Check sheet for the modelled part. Datum: model origin and axes. Units: mm. Give positions to 0.01 mm unless a question says otherwise; leave off trailing zeros. Write each loop counter-clockwise with the first axis right and the second up, starting at its lowest first coordinate (ties: lowest second). Pieces come first, ordered by that corner, then holes. Notation, with made-up numbers: (36, -5.5) -> (62, -5.5) arc R16 ccw to (62, 15.5) -> close; hole circle Ø2 at (64, 48). An arc over 180 degrees is marked (long way). Return JSON: item names as keys, results as strings.
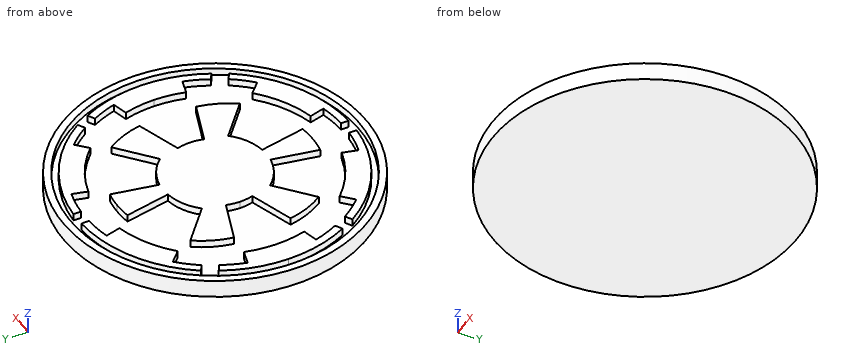
from build123d import *

# Parameters (mm, degrees)
F2_R     = 53.34
F3_DEPTH = 6.35
F0_R     = 50.8
F4_DEPTH = 2.54
F5_DEPTH = 2.54


with BuildPart() as f3:
    # F2 (on Top) → F3 (new body)
    with BuildSketch(Plane.XY):
        Circle(F2_R)
    extrude(amount=-F3_DEPTH)

    # F0 (on Top) → F4 (cut)
    with BuildSketch(Plane.XY):
        Circle(F0_R)
    extrude(amount=-F4_DEPTH, mode=Mode.SUBTRACT)

    # F1 (on Top) → F5 (join)
    with BuildSketch(Plane.XY):
        with BuildLine():
            ThreePointArc((-43.063388, 21.784679), (-46.942873, 11.197957), (-48.26, 0))
            ThreePointArc((-48.26, 0), (-46.942873, -11.197957), (-43.063388, -21.784679))
            Line((-43.063388, -21.784679), (-40.692139, -20.398091))
            ThreePointArc((-40.692139, -20.398091), (-42.512578, -16.297657), (-43.915142, -12.036159))
            Line((-43.915142, -12.036159), (-38.702908, -10.612585))
            ThreePointArc((-38.702908, -10.612585), (-39.772793, -5.354158), (-40.13156, 0))
            ThreePointArc((-40.13156, 0), (-39.772793, 5.354158), (-38.702908, 10.612585))
            Line((-38.702908, 10.612585), (-43.915142, 12.036159))
            ThreePointArc((-43.915142, 12.036159), (-42.512578, 16.297657), (-40.692139, 20.398091))
            Line((-40.692139, 20.398091), (-43.063388, 21.784679))
        make_face()
        with BuildLine():
            Line((-38.165818, -25.239456), (-40.531515, -26.604988))
            ThreePointArc((-40.531515, -26.604988), (-24.179309, -42.023686), (-2.631168, -48.411839))
            Line((-2.631168, -48.411839), (-2.631168, -45.742772))
            ThreePointArc((-2.631168, -45.742772), (-7.132062, -45.269114), (-11.555377, -44.311676))
            Line((-11.555377, -44.311676), (-10.181512, -39.106512))
            ThreePointArc((-10.181512, -39.106512), (-20.139594, -35.033973), (-28.670142, -28.478157))
            Line((-28.670142, -28.478157), (-32.500429, -32.26304))
            ThreePointArc((-32.500429, -32.26304), (-35.517393, -28.899884), (-38.165818, -25.239456))
        make_face()
        with BuildLine():
            Line((-2.71646, -18.05863), (-5.79492, -33.915079))
            ThreePointArc((-5.79492, -33.915079), (-2.907863, -34.283495), (0, -34.406594))
            ThreePointArc((0, -34.406594), (2.907863, -34.283495), (5.79492, -33.915079))
            Line((5.79492, -33.915079), (2.71646, -18.05863))
            ThreePointArc((2.71646, -18.05863), (8.779304, -16.013029), (13.764323, -12.001529))
            Line((13.764323, -12.001529), (25.921796, -22.591443))
            ThreePointArc((25.921796, -22.591443), (29.145002, -16.549346), (31.013678, -9.961172))
            Line((31.013678, -9.961172), (15.781759, -4.649021))
            ThreePointArc((15.781759, -4.649021), (16.283782, -2.348563), (16.452274, 0))
            ThreePointArc((16.452274, 0), (16.283782, 2.348563), (15.781759, 4.649021))
            Line((15.781759, 4.649021), (31.013678, 9.961172))
            ThreePointArc((31.013678, 9.961172), (29.145002, 16.549346), (25.921796, 22.591443))
            Line((25.921796, 22.591443), (13.764323, 12.001529))
            ThreePointArc((13.764323, 12.001529), (8.779304, 16.013029), (2.71646, 18.05863))
            Line((2.71646, 18.05863), (5.79492, 33.915079))
            ThreePointArc((5.79492, 33.915079), (2.907863, 34.283495), (0, 34.406594))
            ThreePointArc((0, 34.406594), (-2.907863, 34.283495), (-5.79492, 33.915079))
            Line((-5.79492, 33.915079), (-2.71646, 18.05863))
            ThreePointArc((-2.71646, 18.05863), (-8.779304, 16.013029), (-13.764323, 12.001529))
            Line((-13.764323, 12.001529), (-25.921796, 22.591443))
            ThreePointArc((-25.921796, 22.591443), (-29.145002, 16.549346), (-31.013678, 9.961172))
            Line((-31.013678, 9.961172), (-15.781759, 4.649021))
            ThreePointArc((-15.781759, 4.649021), (-16.283782, 2.348563), (-16.452274, 0))
            ThreePointArc((-16.452274, 0), (-16.283782, -2.348563), (-15.781759, -4.649021))
            Line((-15.781759, -4.649021), (-31.013678, -9.961172))
            ThreePointArc((-31.013678, -9.961172), (-29.145002, -16.549346), (-25.921796, -22.591443))
            Line((-25.921796, -22.591443), (-13.764323, -12.001529))
            ThreePointArc((-13.764323, -12.001529), (-8.779304, -16.013029), (-2.71646, -18.05863))
        make_face()
        with BuildLine():
            Line((2.631168, -45.742772), (2.631168, -48.411839))
            ThreePointArc((2.631168, -48.411839), (24.179309, -42.023686), (40.531515, -26.604988))
            Line((40.531515, -26.604988), (38.165818, -25.239456))
            ThreePointArc((38.165818, -25.239456), (35.517393, -28.899884), (32.500429, -32.26304))
            Line((32.500429, -32.26304), (28.670142, -28.478157))
            ThreePointArc((28.670142, -28.478157), (20.139594, -35.033973), (10.181512, -39.106512))
            Line((10.181512, -39.106512), (11.555377, -44.311676))
            ThreePointArc((11.555377, -44.311676), (7.132062, -45.269114), (2.631168, -45.742772))
        make_face()
        with BuildLine():
            ThreePointArc((40.13156, 0), (39.772793, -5.354158), (38.702908, -10.612585))
            Line((38.702908, -10.612585), (43.915142, -12.036159))
            ThreePointArc((43.915142, -12.036159), (42.512578, -16.297657), (40.692139, -20.398091))
            Line((40.692139, -20.398091), (43.063388, -21.784679))
            ThreePointArc((43.063388, -21.784679), (46.942873, -11.197957), (48.26, 0))
            ThreePointArc((48.26, 0), (46.942873, 11.197957), (43.063388, 21.784679))
            Line((43.063388, 21.784679), (40.692139, 20.398091))
            ThreePointArc((40.692139, 20.398091), (42.512578, 16.297657), (43.915142, 12.036159))
            Line((43.915142, 12.036159), (38.702908, 10.612585))
            ThreePointArc((38.702908, 10.612585), (39.772793, 5.354158), (40.13156, 0))
        make_face()
        with BuildLine():
            ThreePointArc((40.531515, 26.604988), (24.179309, 42.023686), (2.631168, 48.411839))
            Line((2.631168, 48.411839), (2.631168, 45.742772))
            ThreePointArc((2.631168, 45.742772), (7.132062, 45.269114), (11.555377, 44.311676))
            Line((11.555377, 44.311676), (10.181512, 39.106512))
            ThreePointArc((10.181512, 39.106512), (20.139594, 35.033973), (28.670142, 28.478157))
            Line((28.670142, 28.478157), (32.500429, 32.26304))
            ThreePointArc((32.500429, 32.26304), (35.517393, 28.899884), (38.165818, 25.239456))
            Line((38.165818, 25.239456), (40.531515, 26.604988))
        make_face()
        with BuildLine():
            ThreePointArc((-2.631168, 48.411839), (-24.179309, 42.023686), (-40.531515, 26.604988))
            Line((-40.531515, 26.604988), (-38.165818, 25.239456))
            ThreePointArc((-38.165818, 25.239456), (-35.517393, 28.899884), (-32.500429, 32.26304))
            Line((-32.500429, 32.26304), (-28.670142, 28.478157))
            ThreePointArc((-28.670142, 28.478157), (-20.139594, 35.033973), (-10.181512, 39.106512))
            Line((-10.181512, 39.106512), (-11.555377, 44.311676))
            ThreePointArc((-11.555377, 44.311676), (-7.132062, 45.269114), (-2.631168, 45.742772))
            Line((-2.631168, 45.742772), (-2.631168, 48.411839))
        make_face()
    extrude(amount=-F5_DEPTH)


solid = f3.part
(1) Thickness scan on L1, parallel to X at y = 22, z = -1; L2, parallel to Y at x = -41, z = -1; L3, parallel to Z at x = 39, y = -19. Record the ranges inside material, lowest first.
Reply:
{"L1": "-48.59 to -45.79, -26.31 to -25.24, -3.48 to 3.48, 25.24 to 26.31, 45.79 to 48.59", "L2": "-34.12 to -29.99, -20.58 to -19.78, -11.24 to 11.24, 19.78 to 20.58, 29.99 to 34.12", "L3": "-6.35 to -2.54"}
(2) Cross-section at D-D on y = 6. Enter the section's corners in (x, z), then the cut area to 3 significant figures.
Reply:
{"outline": "(-53, -6.35) -> (53, -6.35) -> (53, 0) -> (50.44, 0) -> (50.44, -2.54) -> (47.89, -2.54) -> (47.89, 0) -> (39.68, 0) -> (39.68, -2.54) -> (19.66, -2.54) -> (19.66, 0) -> (-19.66, 0) -> (-19.66, -2.54) -> (-39.68, -2.54) -> (-39.68, 0) -> (-47.89, 0) -> (-47.89, -2.54) -> (-50.44, -2.54) -> (-50.44, 0) -> (-53, 0) -> close", "area": "558 mm^2"}
(3) Cross-section at C-C on x = 19. Enter the section's corners in (y, z).
Reply:
{"outline": "(-49.84, -6.35) -> (49.84, -6.35) -> (49.84, 0) -> (47.11, 0) -> (47.11, -2.54) -> (44.61, -2.54) -> (44.61, 0) -> (35.66, 0) -> (35.66, -2.54) -> (16.56, -2.54) -> (16.56, 0) -> (5.77, 0) -> (5.77, -2.54) -> (-5.77, -2.54) -> (-5.77, 0) -> (-16.56, 0) -> (-16.56, -2.54) -> (-35.66, -2.54) -> (-35.66, 0) -> (-44.61, 0) -> (-44.61, -2.54) -> (-47.11, -2.54) -> (-47.11, 0) -> (-49.84, 0) -> close"}
(4) Cross-section at A-A on z = -1. State how many separate pieces and enclosed holes the cut face has, then the cut area to 3 significant figures.
Reply:
{"separate pieces": "8", "enclosed holes": "1", "area": "4,220 mm^2"}
(5) Depth check by flat-ended pin: pin 1 Ø0.8 at (y, z) = (-47.5, -1.5) entering from -X; pin 2 Ø0.8 at (y, z) = (47, -1) entering from -X; pin 3 Ø10 at (x, y) = (9.5, -23) entering from +Z. Enter the tip coordinate at first touch or a pass-through.
Reply:
{"pin 1": "x = -25.03", "pin 2": "x = -25.95", "pin 3": "z = -2.54"}
(6) Cross-section at B-B on y = -36. Enter the section's corners in (x, z), then the cut area to 3 significant figures.
Reply:
{"outline": "(-39.36, -6.35) -> (39.36, -6.35) -> (39.36, 0) -> (35.84, 0) -> (35.84, -2.54) -> (32.48, -2.54) -> (32.48, 0) -> (18.36, 0) -> (18.36, -2.54) -> (-18.36, -2.54) -> (-18.36, 0) -> (-32.48, 0) -> (-32.48, -2.54) -> (-35.84, -2.54) -> (-35.84, 0) -> (-39.36, 0) -> close", "area": "390 mm^2"}
